For this review, take the finished solid that the model builds, in its own axes (mm). A direction names the side the tool comes from. Round coordinates to 2 decimals unless told otherwise and drop trailing zeros. Order: outer loops, then holes, each group sorted by start corner. A loop starts at its lowest first (then second) coordinate and runs counter-clockwise, first axis right, second up. Notation, with made-up numbers: M 58,56 L 74,56 A24 cw 74,80 Z; hole C 37.5,-39 d6. An arc over 180 degrees is marked long. Put each result on its own line as item: value.
from build123d import *

# Parameters (mm, degrees)
SKETCH1_W                    = 482.6
SKETCH1_H                    = 420.37
BASE_FLANGE1_DEPTH           = 3.175
EDGE_FLANGE1_STRIP_W         = 14.7
EDGE_FLANGE1_STRIP_H         = 3.175
EDGE_FLANGE1_STRIP_CUT_DEPTH = 482.6
EDGE_FLANGE1_DEPTH           = 482.6
EDGE_FLANGE3_DEPTH           = 215.9


# Sheet-metal steps are written as plain solids
with BuildPart() as part:
    # Sketch1 → Base-Flange1 (new body)
    with BuildSketch(Plane.XY):
        Rectangle(SKETCH1_W, SKETCH1_H)
    extrude(amount=-BASE_FLANGE1_DEPTH)

    # Edge-Flange1 strip (across the edge) → Edge-Flange1 strip cut (cut)
    with BuildSketch(Plane(origin=(-241.3, -210.185, 0), x_dir=(0, 1, 0), z_dir=(1, 0, 0))):
        with Locations((-3.175, -1.5875)):
            Rectangle(EDGE_FLANGE1_STRIP_W, EDGE_FLANGE1_STRIP_H)
    extrude(amount=EDGE_FLANGE1_STRIP_CUT_DEPTH, mode=Mode.SUBTRACT)

    # Edge-Flange1 section (across the edge) → Edge-Flange1 (add)
    with BuildSketch(Plane(origin=(-241.3, -210.185, 0), x_dir=(0, 1, 0), z_dir=(1, 0, 0))):
        with BuildLine():
            Line((0, 1), (0, 9.525))
            Line((0, 9.525), (3.175, 9.525))
            Line((3.175, 9.525), (3.175, 1))
            ThreePointArc((3.175, 1), (3.467893219, 0.292893219), (4.175, 0))
            Line((4.175, 0), (4.175, -3.175))
            ThreePointArc((4.175, -3.175), (1.222829189, -1.952170811), (0, 1))
        make_face()
    extrude(amount=EDGE_FLANGE1_DEPTH)

    # Edge-Flange3 section (across the edge) → Edge-Flange3 (add)
    with BuildSketch(Plane(origin=(242.57, 210.185, -3.175), x_dir=(-1, 0, 0), z_dir=(0, -1, 0))):
        with BuildLine():
            Line((-3.175, 1), (-3.175, 10.120953567))
            Line((-3.175, 10.120953567), (0, 10.120953567))
            Line((0, 10.120953567), (0, 1))
            ThreePointArc((0, 1), (0.292893219, 0.292893219), (1, 0))
            Line((1, 0), (1.27, 0))
            Line((1.27, 0), (1.27, -3.175))
            Line((1.27, -3.175), (1, -3.175))
            ThreePointArc((1, -3.175), (-1.952170811, -1.952170811), (-3.175, 1))
        make_face()
    edge_flange3 = extrude(amount=EDGE_FLANGE3_DEPTH)

    # Mirror2: Edge-Flange3 across plane
    add(edge_flange3.mirror(Plane(origin=(0, 0, 0), x_dir=(0, 0, 1), z_dir=(1, 0, 0))))


solid = part.part
(1) Add section A-A on z = -9.5. Give the boundary of the cut face in (x, y) (3 decimals).
A:
outline: M -245.745,-5.715 L -242.57,-5.715 L -242.57,210.185 L -245.745,210.185 Z; M 242.57,-5.715 L 245.745,-5.715 L 245.745,210.185 L 242.57,210.185 Z
(2) Draft analysis for pull direction Y (two halves, no side actions). For faces 1 (the face through (1, 210.185, -2)), 2 (the face through (-241.3, -107, -1)), state which applies: released by +Y, released by -Y, zero draft, split by the parting line, or undercut.
A:
face 1: released by +Y
face 2: zero draft
(3) Add section C-C on y = 41. Give the boundary of the cut face in (x, z) (3 decimals).
A:
outline: M -245.745,-13.296 L -242.57,-13.296 L -242.57,-4.175 A1 cw -241.57,-3.175 L 241.57,-3.175 A1 cw 242.57,-4.175 L 242.57,-13.296 L 245.745,-13.296 L 245.745,-4.175 A4.175 ccw 241.57,0 L -241.57,0 A4.175 ccw -245.745,-4.175 Z
(4) Insertion check: pin 1 Ø8 at (y, z) = (-73, -6.5) entering from +X; pin 2 Ø10 at (x, y) = (-42, -43.5) entering from -Z (3 decimals); pin 3 Ø2 at (x, z) = (242.5, -10) entering from -Y (3 decimals); pin 4 Ø1 at (x, z) = (68.5, -4) entering from -Y. Each pin has a flat end and moves straight along its axis. Give the tip position at first contact, or say it passes through.
A:
pin 1: stops at x = 241.3
pin 2: stops at z = -3.175
pin 3: stops at y = -5.715
pin 4: passes through
(5) To check wall thickness, follow L1, parallel to X at y = -2, z = -4.25 (3 decimals); L2, parallel to Z at x = 19, y = 61 (3 decimals); L3, parallel to Y at x = -81.5, z = 6.5 (3 decimals). State the ranges of each line that lie inside material, in increasing order.
A:
L1: x = -245.745 to -242.57, 242.57 to 245.745
L2: z = -3.175 to 0
L3: y = -210.185 to -207.01
(6) Add section B-B on x = 111.5. Give the boundary of the cut face in (y, z) (3 decimals).
A:
outline: M -210.185,1 A4.175 ccw -206.01,-3.175 L 210.185,-3.175 L 210.185,0 L -206.01,0 A1 cw -207.01,1 L -207.01,9.525 L -210.185,9.525 Z
(7) Add section D-D on y = -149. Give the boundary of the cut face in (x, z) (3 decimals).
A:
outline: M -241.3,-3.175 L 241.3,-3.175 L 241.3,0 L -241.3,0 Z
(8) For faces 3 (the face through (-3, 5, -3.175)), 4 (the face through (3, 5, 0)), 5 (the face through (241.3, -107, -1)), list the 3-axis set-ups (+Z, -Z, +X, -X, +Y, -Y) from which the entire face can be reached by the end or side of a thin tool; tool diameter is ignored.
A:
face 3: -Z, +Y, -Y
face 4: +Z, +X, -X, +Y
face 5: +Z, -Z, +X, -Y
